For this review, take the finished solid that the model builds, in its own axes (mm). Give positions to 0.01 mm unless a question says otherwise; leave off trailing zeros. Write each loop counter-clockwise with the first axis right and the second up, starting at its lowest first coordinate (ties: lowest second). Pieces come first, ordered by that corner, then holes. Notation, with made-up numbers: M -9,4 L 49,4 A20 cw 49,23 Z; hole C 33,20.25 d6. An arc over 180 degrees is marked long. Use one line per item in the form item = value. Start each with the question number.
Q1. Consider section C-C on z = 13.5. Give the number of separate pieces and of enclosed holes in the cut face, and give its area (3 significant figures).
Q2. Consider section B-B on x = 125.5. Write out the cut boundary in (y, z).
Q3. Clearance check with flat-ended pins moving along their axes: pin 1 Ø9.5 at (x, z) = (1028.5, 11) entering from +Y; pin 2 Ø5.5 at (y, z) = (287.5, 12) entering from -X; pin 3 Ø9.5 at (y, z) = (319.5, 13.5) entering from +X. State where each tip first meets the part, or that it passes through.
Q4. Consider section D-D on x = -135. Write out the cut boundary in (y, z).
Q5. Consider section A-A on y = 12.5. Write out the cut boundary in (x, z), and give its area (3 significant figures).
Q6. Mouldability with a two-part tool opening along X and no side actions: class faces 1 (the flat face through (-137, -40, 0)), 2 (the cylindrical face through (4.12, -78.955, 9.392)) as released by +X, released by -X, zero draft, split by the parting line, or undercut.
Q7. For probe 1 along X at (y, z) = (15, 11.75); probe 2 along Y at (x, z) = (-464, 15.5); probe 3 along Y at (x, z) = (-343, 7.5), list the stretches that pass through material, from the lowest coordinate up. Write a range as [from, to].
Autodesk Inventor part; units mm, degrees
ref_plane "YZ Plane" through (0, 0, 0) normal (1, 0, 0) x (0, 1, 0)
ref_plane "XZ Plane" through (0, 0, 0) normal (0, 1, 0) x (-1, 0, 0)
ref_plane "XY Plane" through (0, 0, 0) normal (0, 0, 1) x (1, 0, 0)
sketch "Sketch1" plane through (0, 0, 0) normal (0, 0, 1) x (1, 0, 0)
  line L0 (-998.1754, 340.1521) -> (1033.8246, 340.1521)
  line L1 (1033.8246, 340.1521) -> (1033.8246, -117.0479)
  line L2 (-998.1754, -117.0479) -> (-998.1754, 340.1521)
  arc A0 (995.7246, -117.0479) -> (-960.0754, -117.0479) centre (17.8246, -12647.7146) ccw
  line L3 (1033.8246, -117.0479) -> (995.7246, -117.0479)
  line L4 (-960.0754, -117.0479) -> (-998.1754, -117.0479)
  point P0 (0, 0)
  dimension "d0" = 2032
  dimension "d1" = 457.2
extrude "Extrusion1" add sketch "Sketch1" along normal blind 19.05
sketch "Sketch2" plane through (0, 0, 19.05) normal (0, 0, 1) x (1, 0, 0)
  line L0 (1033.8246, 340.1521) -> (-998.1754, 340.1521)
  line L1 (-998.1754, -117.0479) -> (-960.0754, -117.0479)
  line L2 (-998.1754, 340.1521) -> (-979.1254, 340.1521)
  line L3 (-979.1254, 340.1521) -> (-979.1254, -117.0479)
  line L4 (-979.1254, -117.0479) -> (-998.1754, -117.0479)
  line L5 (-998.1754, -117.0479) -> (-998.1754, 340.1521)
  line L6 (1033.8246, -117.0479) -> (1033.8246, 340.1521)
  line L7 (1033.8246, 340.1521) -> (1014.7746, 340.1521)
  line L8 (1014.7746, 340.1521) -> (1014.7746, -117.0479)
  line L9 (1014.7746, -117.0479) -> (1033.8246, -117.0479)
  line L10 (1033.8246, -117.0479) -> (1033.8246, 340.1521)
  line L11 (-998.1754, 340.1521) -> (-998.1754, -117.0479)
  line L12 (-998.1754, 263.9521) -> (-979.1254, 263.9521)
  line L13 (1014.7746, 263.9521) -> (1033.8246, 263.9521)
  line L14 (-998.1754, 187.7521) -> (-979.1254, 187.7521)
  line L15 (1014.7746, 187.7521) -> (1033.8246, 187.7521)
  line L16 (-998.1754, 111.5521) -> (-979.1254, 111.5521)
  line L17 (1014.7746, 111.5521) -> (1033.8246, 111.5521)
  line L18 (-998.1754, 35.3521) -> (-979.1254, 35.3521)
  line L19 (1014.7746, 35.3521) -> (1033.8246, 35.3521)
  line L20 (1033.8246, -40.8479) -> (1014.7746, -40.8479)
  line L21 (-979.1254, -40.8479) -> (-998.1754, -40.8479)
  point P0 (0, 0)
  dimension "d7" = 19.05
  dimension "d8" = 19.05
extrude "Extrusion2" cut sketch "Sketch2" against normal blind 19.05 contours L6 L13 L8 L0 | L3 L12 L5 L0 | L6 L17 L8 L15 | L3 L16 L5 L14 | L6 L20 L8 L19 | L3 L21 L5 L18
sketch "Sketch4" plane through (0, 0, 19.05) normal (0, 0, 1) x (1, 0, 0)
  line L0 (-845.7754, -40.8479) -> (-845.7754, -59.8979)
  line L1 (-998.1754, 111.5521) -> (-998.1754, 35.3521)
  line L2 (-642.5754, -40.8479) -> (-642.5754, -59.8979)
  line L3 (-540.9754, -40.8479) -> (-540.9754, -59.8979)
  line L4 (-337.7754, -40.8479) -> (-337.7754, -59.8979)
  line L5 (-236.1754, -40.8479) -> (-236.1754, -59.8979)
  line L6 (-32.9754, -40.8479) -> (-32.9754, -59.8979)
  line L7 (68.6246, -40.8479) -> (68.6246, -59.8267)
  line L8 (271.8246, -40.8479) -> (271.8246, -59.8267)
  line L9 (373.4246, -40.8479) -> (373.4246, -59.8979)
  line L10 (576.6246, -40.8479) -> (576.6246, -59.8979)
  line L11 (678.2246, -40.8479) -> (678.2246, -59.8979)
  line L12 (881.4246, -40.8479) -> (881.4246, -59.8979)
  arc A0 (995.7246, -117.0479) -> (-960.0754, -117.0479) centre (17.8246, -12647.7146) ccw
  line L13 (-998.1754, -40.8479) -> (-998.1754, -117.0479)
  line L14 (1014.7746, 340.1521) -> (-979.1254, 340.1521)
  line L15 (1014.7746, 340.1521) -> (1014.7746, 263.9521)
  line L16 (-979.1254, 340.1521) -> (1014.7746, 340.1521)
  line L17 (-845.7754, -40.8479) -> (-642.5754, -40.8479)
  line L18 (-845.7754, -59.8979) -> (-642.5754, -59.8979)
  line L19 (-540.9754, -59.8979) -> (-337.7754, -59.8979)
  line L20 (-540.9754, -40.8479) -> (-337.7754, -40.8479)
  line L21 (-236.1754, -40.8479) -> (-32.9754, -40.8479)
  line L22 (68.6246, -40.8479) -> (271.8246, -40.8479)
  line L23 (373.4246, -59.8979) -> (576.6246, -59.8979)
  line L24 (678.2246, -59.8979) -> (881.4246, -59.8979)
  line L25 (373.4246, -40.8479) -> (576.6246, -40.8479)
  line L26 (678.2246, -40.8479) -> (881.4246, -40.8479)
  line L27 (-236.1754, -59.8979) -> (-32.9754, -59.8979)
  line L28 (68.6246, -59.8267) -> (271.8246, -59.8267)
  point P0 (0, 0)
  dimension "d18" = 152.4
  dimension "d19" = 203.2
  dimension "d26" = 457.2
  dimension "d27" = 203.2
  dimension "d28" = 101.6
  dimension "d29" = 203.2
  dimension "d30" = 101.6
  dimension "d31" = 101.6
  dimension "d32" = 101.6
  dimension "d33" = 203.2
  dimension "d34" = 203.2
  dimension "d35" = 203.2
extrude "Extrusion4" cut sketch "Sketch4" against normal blind 25.4
sketch "Sketch5" plane through (0, 0, 19.05) normal (0, 0, 1) x (1, 0, 0)
  line L0 (-833.0754, 302.0521) -> (995.7246, 302.0521)
  line L1 (995.7246, 302.0521) -> (995.7246, -15.4479)
  line L2 (995.7246, -15.4479) -> (-833.0754, -15.4479)
  line L3 (-833.0754, -15.4479) -> (-833.0754, 302.0521)
  line L4 (1014.7746, 340.1521) -> (-979.1254, 340.1521)
  line L5 (1033.8246, 187.7521) -> (1033.8246, 263.9521)
  point P0 (0, 0)
  dimension "d36" = 355.6
  dimension "d37" = 38.1
  dimension "d38" = 38.1
  dimension "d39" = 1828.8
extrude "Extrusion5" cut sketch "Sketch5" against normal blind 25.4
properties part number "front" material "Wood (Birch)"
Working result:
q1.separate_pieces = 1
q1.enclosed_holes = 7
q1.area = 267,000 mm²
q2.outline = M -79.41,0 L -59.83,0 L -59.83,19.05 L -79.41,19.05 Z; M -40.85,0 L -15.45,0 L -15.45,19.05 L -40.85,19.05 Z; M 302.05,0 L 340.15,0 L 340.15,19.05 L 302.05,19.05 Z
q3.pin_1 = 263.95
q3.pin_2 = -979.13
q3.pin_3 = 1014.77
q4.outline = M -79.88,0 L -59.9,0 L -59.9,19.05 L -79.88,19.05 Z; M -40.85,0 L -15.45,0 L -15.45,19.05 L -40.85,19.05 Z; M 302.05,0 L 340.15,0 L 340.15,19.05 L 302.05,19.05 Z
q5.outline = M -979.13,0 L -833.08,0 L -833.08,19.05 L -979.13,19.05 Z; M 995.72,0 L 1014.77,0 L 1014.77,19.05 L 995.72,19.05 Z
q5.area = 3,150 mm²
q6.face_1 = zero draft
q6.face_2 = undercut
q7.probe_1 = [-979.13, -833.08], [995.72, 1014.77]
q7.probe_2 = [-88.19, -59.9], [-40.85, -15.45], [302.05, 340.15]
q7.probe_3 = [-84.13, -59.9], [-40.85, -15.45], [302.05, 340.15]
